Geometry check sheet. Reference: drawing and pictorial views, mm from the part's lowest x, y, z. A direction names the side the tool comes from. Give positions to 0.01 mm unless a question says otherwise; leave off trailing zeros. Write each loop counter-clockwise with the first axis right and the second up, starting at its lowest first coordinate (ties: lowest second). Pieces come first, ordered by that corner, then holes.
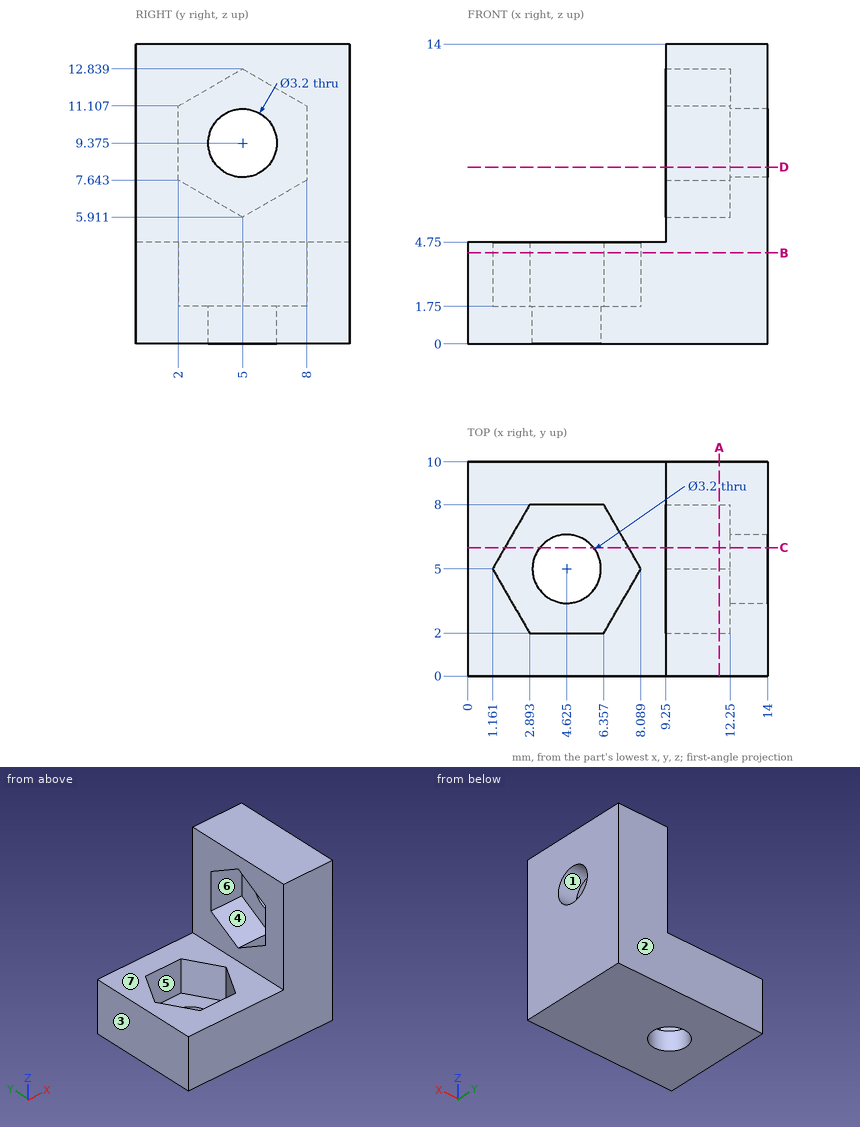
Item 1: Scan lines: line 1 along Y through (x, z) = (13.25, 9.5) (3 decimals); line 2 along Z through (x, y) = (13.15, 5) (3 decimals); line 3 along Z through (x, y) = (8.75, 1). Record each from-to range of solid material in increasing order.
Answer key:
line 1: y = 0 to 3.405, 6.595 to 10
line 2: z = 0 to 7.775, 10.975 to 14
line 3: z = 0 to 4.75
Item 2: Sectioned sample at D-D on z = 8.25. Record the cut outline in (x, y), then the cut area to 3 significant figures.
Answer key:
outline: (9.25, 0) - (14, 0) - (14, 3.86) - (12.25, 3.86) - (12.25, 2) - (9.25, 2) - close; (9.25, 8) - (12.25, 8) - (12.25, 6.14) - (14, 6.14) - (14, 10) - (9.25, 10) - close
area: 25.5 mm2
Item 3: Sectioned sample at A-A on x = 11.75. Record the cut outline in (y, z).
Answer key:
outline: (0, 0) - (10, 0) - (10, 14) - (0, 14) - close; hole (2, 7.64) - (5, 5.91) - (8, 7.64) - (8, 11.11) - (5, 12.84) - (2, 11.11) - close
Item 4: Sectioned sample at B-B on z = 4.25. Record the cut outline in (x, y).
Answer key:
outline: (0, 0) - (14, 0) - (14, 10) - (0, 10) - close; hole (1.16, 5) - (2.89, 2) - (6.36, 2) - (8.09, 5) - (6.36, 8) - (2.89, 8) - close
Item 5: Set-up check for the marked faces 5, 6 and 7: record each of +Z, -Z, +X, -X, +Y, -Y from which the full face is reachable in a straight line by a thin tool's end or side.
Answer key:
face 5: +Z
face 6: -X
face 7: +Z, -X, +Y, -Y
Item 6: Release check for a two-part mould opening along Y. For the marked faces 1, 2, 3 and 4 record: released by +Y, released by -Y, zero draft, split by the parting line, or undercut.
Answer key:
face 1: undercut
face 2: released by +Y
face 3: zero draft
face 4: undercut
Item 7: Sectioned sample at C-C on y = 6. Record the cut outline in (x, z).
Answer key:
outline: (0, 0) - (3.38, 0) - (3.38, 1.75) - (1.74, 1.75) - (1.74, 4.75) - (0, 4.75) - close; (5.87, 0) - (14, 0) - (14, 8.13) - (12.25, 8.13) - (12.25, 6.49) - (9.25, 6.49) - (9.25, 4.75) - (7.51, 4.75) - (7.51, 1.75) - (5.87, 1.75) - close; (9.25, 12.26) - (12.25, 12.26) - (12.25, 10.62) - (14, 10.62) - (14, 14) - (9.25, 14) - close
Item 8: Depth check by flat-ended pin: pin 1 (3 mm diameter, centred on y = 5, z = 10, fed in from -X); pin 2 (3.5 mm diameter, centred on x = 4.625, y = 5, fed in from +Z); pin 3 (3 mm diameter, centred on y = 3.5, z = 10.5, fed in from -X). Enter the tip coordinate at first touch or a pass-through.
Answer key:
pin 1: stops at x = 12.25
pin 2: stops at z = 1.75
pin 3: stops at x = 9.25
